```python
from build123d import *

# Parameters (mm, degrees)
F0_R           = 7
F0_R_2         = 50
F0_W           = 200
F0_H           = 40
F1_DEPTH       = 40
F2_D           = 12.1
F3_DEPTH       = 300
F5_D           = 17.5
F5_CBORE_D     = 31.5
F5_CBORE_DEPTH = 20
F7_DEPTH       = 12.5


with BuildPart() as f1:
    # F0 (on Front) → F1 (new body)
    with BuildSketch(Plane.XZ):
        with BuildLine():
            ThreePointArc((-100, 0), (0, -100), (100, 0))
            ThreePointArc((100, 0), (0, 100), (-100, 0))
        make_face()
        with Locations((0, -72)):
            Circle(F0_R, mode=Mode.SUBTRACT)
        with Locations((-72, 0)):
            Circle(F0_R, mode=Mode.SUBTRACT)
        Circle(F0_R_2, mode=Mode.SUBTRACT)
        with Locations((72, 0)):
            Circle(F0_R, mode=Mode.SUBTRACT)
        with Locations((0, 72)):
            Circle(F0_R, mode=Mode.SUBTRACT)
        with BuildLine():
            Line((100, -160), (100, 0))
            ThreePointArc((100, 0), (0, -100), (-100, 0))
            Line((-100, 0), (-100, -160))
            Line((-100, -160), (100, -160))
        make_face()
        with Locations((0, -180)):
            Rectangle(F0_W, F0_H)
        with Locations((0, 72)):
            Circle(F0_R)
        with Locations((72, 0)):
            Circle(F0_R)
        with Locations((0, -72)):
            Circle(F0_R)
        with Locations((-72, 0)):
            Circle(F0_R)
    extrude(amount=F1_DEPTH)

    # F2 (through all)
    with Locations(Plane(origin=(0, 0, 0), x_dir=(1, 0, 0), z_dir=(0, 1, 0))):
        with Locations((-72, 0), (0, 72), (72, 0), (0, -72)):
            Hole(F2_D / 2)

    # F0 (on Front) → F3 (join)
    with BuildSketch(Plane.XZ):
        with Locations((0, -180)):
            Rectangle(F0_W, F0_H)
    extrude(amount=F3_DEPTH)

    # F5 (through all)
    with Locations(Plane.XY.offset(-160)):
        with Locations((60, -260), (-60, -260), (60, -140), (-60, -140)):
            CounterBoreHole(F5_D / 2, F5_CBORE_D / 2, F5_CBORE_DEPTH)

    # F6 (on Right) → F7 (join, symmetric)
    with BuildSketch(Plane.YZ):
        Polygon((-40, -160), (-40, -100), (-100, -160), align=None)
    extrude(amount=F7_DEPTH, both=True)


solid = f1.part
```
Part model, mm, in its own coordinate system. A direction names the side the tool comes from. Round coordinates to 2 decimals unless told otherwise and drop trailing zeros. Write each loop counter-clockwise with the first axis right and the second up, starting at its lowest first coordinate (ties: lowest second). Pieces come first, ordered by that corner, then holes. Notation, with made-up numbers: (76, 69.25) -> (82, 69.25) arc R24 cw to (82, 97.25) -> close; hole circle Ø1 at (-36, -12). An arc over 180 degrees is marked (long way). Return JSON: item names as keys, results as strings. Group by question number.
Q1. Pin check, flat tips, straight feed: pin 1 (19.5 mm diameter, centred on x = 0, z = 72, fed in from -Y); pin 2 (5 mm diameter, centred on x = 24, y = -43, fed in from +Z). Stop position of each tip, or through.
Q2. Which spindle directions (+Z, -Z, +X, -X, +Y, -Y) get a long thin tool onto all of the face, cutting with end or side? Do faces 5 (the cylindrical face through (2.199, -19.72, 99.976)), 6 (the flat face through (-12.5, -57, -143)), 7 (the flat face through (-53, -147, -180)). Say none if no direction does.
Q3. Saw through at B-B on y = -30. Write the cut outline in (x, z), plus the area to 3 significant figures.
Q4. Mould opens along X. For faces 1 (the flat face through (12.5, -57, -143)), 2 (the flat face through (67, -147, -180)), 3 (the flat face through (-1, -40, -57)), 4 (the cylindrical face through (0.79, -20.28, -78)) say: pulls with the +X half, pulls with the -X half, needs draft (parallel to the pull), parting line crosses it, or undercut.
Q5. Saw through at A-A on z = -72. Write the cut outline in (x, y).
Q6. Probe L1, parallel to Y at x = -60, z = -170.75; L2, parallel to Y at x = -60, z = -185.25; L3, parallel to X at y = -11, z = -72. List the from-to ranges inside material, lowest first. Write a range as [from, to].
Q7. Saw through at D-D on y = -140. Write the cut outline in (x, z), plus the area to 3 significant figures.
Q8. Saw through at C-C on x = -60. Write the cut outline in (y, z), plus the area to 3 significant figures.
Answer:
{
 "1": {"pin 1": "y = -40", "pin 2": "z = -160"},
 "2": {"face 5": "+Z, +Y, -Y", "face 6": "+Z, -X, -Y", "face 7": "+Z"},
 "3": {"outline": "(-100, -200) -> (100, -200) -> (100, 0) arc R100 ccw to (-100, 0) -> close; hole circle Ø12.1 at (-72, 0); hole circle Ø100 at (0, 0); hole circle Ø12.1 at (0, -72); hole circle Ø12.1 at (0, 72); hole circle Ø12.1 at (72, 0)", "area": "47,400 mm2"},
 "4": {"face 1": "pulls with the +X half", "face 2": "undercut", "face 3": "needs draft", "face 4": "undercut"},
 "5": {"outline": "(-100, -40) -> (-6.05, -40) -> (-6.05, 0) -> (-100, 0) -> close; (6.05, -40) -> (100, -40) -> (100, 0) -> (6.05, 0) -> close"},
 "6": {"L1": "[-300, -275.75], [-244.25, -155.75], [-124.25, 0]", "L2": "[-300, -268.75], [-251.25, -148.75], [-131.25, 0]", "L3": "[-100, -6.05], [6.05, 100]"},
 "7": {"outline": "(-100, -200) -> (-68.75, -200) -> (-68.75, -180) -> (-75.75, -180) -> (-75.75, -160) -> (-100, -160) -> close; (-51.25, -200) -> (51.25, -200) -> (51.25, -180) -> (44.25, -180) -> (44.25, -160) -> (-44.25, -160) -> (-44.25, -180) -> (-51.25, -180) -> close; (68.75, -200) -> (100, -200) -> (100, -160) -> (75.75, -160) -> (75.75, -180) -> (68.75, -180) -> close", "area": "6,040 mm2"},
 "8": {"outline": "(-300, -200) -> (-268.75, -200) -> (-268.75, -180) -> (-275.75, -180) -> (-275.75, -160) -> (-300, -160) -> close; (-251.25, -200) -> (-148.75, -200) -> (-148.75, -180) -> (-155.75, -180) -> (-155.75, -160) -> (-244.25, -160) -> (-244.25, -180) -> (-251.25, -180) -> close; (-131.25, -200) -> (0, -200) -> (0, 80) -> (-40, 80) -> (-40, -160) -> (-124.25, -160) -> (-124.25, -180) -> (-131.25, -180) -> close", "area": "19,600 mm2"}
}
